Build history of the part. All positions in model axes, mm. Face numbers are marked on the shaded views. A direction names the side the tool comes from. Round coordinates to 2 decimals unless told otherwise and drop trailing zeros. Write each loop counter-clockwise with the first axis right and the second up, starting at its lowest first coordinate (ties: lowest second). Pieces come first, ordered by that corner, then holes. Notation, with made-up numbers: (76.5, 60) - (83.5, 60) arc R28 cw to (83.5, 87) - close; hole circle Ø7 at (-14, -15). An arc over 180 degrees is marked (long way). Write each question's results on one line, items separated by ' | '.
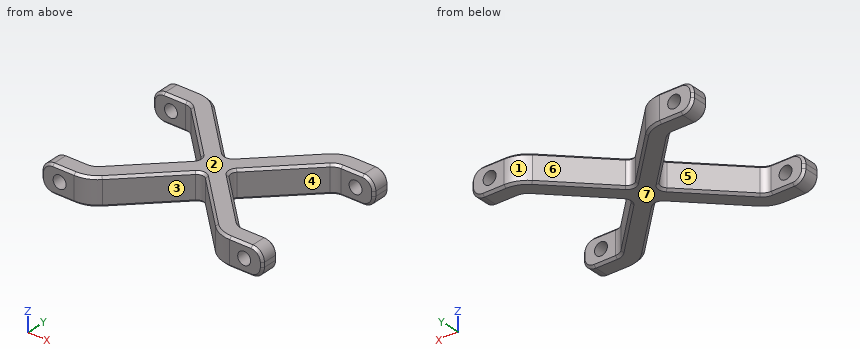
from build123d import *

# Parameters (mm, degrees)
EXTRUIR_L_MINA1_DEPTH    = 6
TALADRO1_D               = 5.6
TALADRO1_DEPTH           = 68
REDONDEO1_R              = 5
REDONDEO1_OF_SIMETR_A1_R = 5
REDONDEO3_R              = 3
CHAFL_N4_SIZE            = 1


# Read off the part's stored shape, not the designer's step: Simetría2
with BuildPart() as part:
    # Croquis1 → Extruir-Lámina1 (new, symmetric)
    with BuildSketch(Plane.XY):
        with BuildLine():
            Line((2.828427125, -2.828427125), (30.192388155, 24.535533906))
            ThreePointArc((30.192388155, 24.535533906), (31.8145049, 25.619397663), (33.727922061, 26))
            Line((33.727922061, 26), (48, 26))
            Line((48, 26), (48, 34))
            Line((48, 34), (33.727922061, 34))
            ThreePointArc((33.727922061, 34), (28.753037441, 33.010433923), (24.535533906, 30.192388155))
            Line((24.535533906, 30.192388155), (-2.828427125, 2.828427125))
            Line((-2.828427125, 2.828427125), (2.828427125, -2.828427125))
        make_face()
    extruir_l_mina1 = extrude(amount=EXTRUIR_L_MINA1_DEPTH, both=True)

    # Taladro1
    with Locations(Plane(origin=(0, 34, 0), x_dir=(1, 0, 0), z_dir=(0, 1, 0))):
        with Locations((40, 0)):
            taladro1 = Hole(TALADRO1_D / 2, depth=TALADRO1_DEPTH)

    # Redondeo1
    redondeo1_edges = [part.edges().sort_by_distance(p)[0] for p in [
        (48, 30, 6),
        (48, 30, -6),
    ]]
    fillet(redondeo1_edges, radius=REDONDEO1_R)

    # Simetría1: Extruir-Lámina1, Taladro1 across plane
    add(extruir_l_mina1.mirror(Plane(origin=(0, 0, 0), x_dir=(0, 0, 1), z_dir=(1, 0, 0))))
    add(taladro1.mirror(Plane(origin=(0, 0, 0), x_dir=(0, 0, 1), z_dir=(1, 0, 0))), mode=Mode.SUBTRACT)

    # Redondeo1 of Simetría1
    redondeo1_of_simetr_a1_edges = [part.edges().sort_by_distance(p)[0] for p in [
        (-48, 30, 6),
        (-48, 30, -6),
    ]]
    fillet(redondeo1_of_simetr_a1_edges, radius=REDONDEO1_OF_SIMETR_A1_R)

    # Simetría2: part across plane


with BuildPart() as part_1:
    add(part.part)
    add(part.part.mirror(Plane.ZX))

    # Redondeo3
    redondeo3_edges = [part_1.edges().sort_by_distance(p)[0] for p in [
        (-5.656854249, 0, 0),
        (5.656854249, 0, 0),
        (0, -5.656854249, 0),
        (0, 5.656854249, 0),
    ]]
    fillet(redondeo3_edges, radius=REDONDEO3_R)

    # Chaflán4
    chafl_n4_edges = [part_1.edges().sort_by_distance(p)[0] for p in [
        (38.363961031, 34, -6),
        (-38.363961031, -26, -6),
        (-31.8145049, -25.619397663, -6),
        (-28.753037441, -33.010433923, 6),
        (-38.363961031, -34, 6),
        (-28.753037441, -33.010433923, -6),
        (-38.363961031, -34, -6),
        (-31.8145049, -25.619397663, 6),
        (-38.363961031, -26, 6),
        (28.753037441, 33.010433923, -6),
        (-48, -26, 0),
        (-46.535533906, -26, 4.535533906),
        (-46.535533906, -26, -4.535533906),
        (-48, -34, 0),
        (-46.535533906, -34, 4.535533906),
        (-46.535533906, -34, -4.535533906),
        (38.363961031, -26, 6),
        (38.363961031, -34, -6),
        (28.753037441, -33.010433923, -6),
        (31.8145049, -25.619397663, 6),
        (31.8145049, -25.619397663, -6),
        (38.363961031, -26, -6),
        (28.753037441, -33.010433923, 6),
        (38.363961031, -34, 6),
        (48, -26, 0),
        (48, -34, 0),
        (38.363961031, 34, 6),
        (46.535533906, -26, 4.535533906),
        (46.535533906, -26, -4.535533906),
        (28.753037441, 33.010433923, 6),
        (46.535533906, -34, 4.535533906),
        (46.535533906, -34, -4.535533906),
        (13.328427125, -18.985281374, 6),
        (13.328427125, -18.985281374, -6),
        (18.985281374, 13.328427125, 6),
        (18.985281374, 13.328427125, -6),
        (18.985281374, -13.328427125, 6),
        (18.985281374, -13.328427125, -6),
        (-18.985281374, 13.328427125, -6),
        (-18.985281374, 13.328427125, 6),
        (-18.985281374, -13.328427125, -6),
        (38.363961031, 26, 6),
        (-18.985281374, -13.328427125, 6),
        (13.328427125, 18.985281374, -6),
        (13.328427125, 18.985281374, 6),
        (-13.328427125, 18.985281374, -6),
        (-13.328427125, -18.985281374, 6),
        (-13.328427125, 18.985281374, 6),
        (0, -6.899494937, -6),
        (0, -6.899494937, 6),
        (31.8145049, 25.619397663, 6),
        (6.899494937, 0, -6),
        (6.899494937, 0, 6),
        (-6.899494937, 0, 6),
        (-6.899494937, 0, -6),
        (0, 6.899494937, 6),
        (0, 6.899494937, -6),
        (-13.328427125, -18.985281374, -6),
        (31.8145049, 25.619397663, -6),
        (38.363961031, 26, -6),
        (48, 26, 0),
        (46.535533906, 26, 4.535533906),
        (46.535533906, 26, -4.535533906),
        (48, 34, 0),
        (46.535533906, 34, 4.535533906),
        (46.535533906, 34, -4.535533906),
        (-31.8145049, 25.619397663, -6),
        (-38.363961031, 26, -6),
        (-28.753037441, 33.010433923, 6),
        (-38.363961031, 34, 6),
        (-38.363961031, 26, 6),
        (-38.363961031, 34, -6),
        (-28.753037441, 33.010433923, -6),
        (-31.8145049, 25.619397663, 6),
        (-48, 26, 0),
        (-48, 34, 0),
        (-46.535533906, 26, 4.535533906),
        (-46.535533906, 26, -4.535533906),
        (-46.535533906, 34, 4.535533906),
        (-46.535533906, 34, -4.535533906),
    ]]
    chamfer(chafl_n4_edges, length=CHAFL_N4_SIZE)


solid = part_1.part
(1) Slice it at A-A, the plane x = 40. Write the cut outline in (y, z).
Worked answers:
outline: (-34, -5) - (-33, -6) - (-27, -6) - (-26, -5) - (-26, -2.8) - (-34, -2.8) - close; (-34, 2.8) - (-26, 2.8) - (-26, 5) - (-27, 6) - (-33, 6) - (-34, 5) - close; (26, -5) - (27, -6) - (33, -6) - (34, -5) - (34, -2.8) - (26, -2.8) - close; (26, 2.8) - (34, 2.8) - (34, 5) - (33, 6) - (27, 6) - (26, 5) - close
(2) Drill centre lines: probe 1 along Z at (x, y) = (-40, 30.75); probe 2 along Y at (x, z) = (36, 4.5); probe 3 along Y at (x, z) = (-24, 0). Where is each one in solid material? Low to high. Write a range as [from, to].
Worked answers:
probe 1: z = [-6, -2.8], [2.8, 6] | probe 2: y = [-34, -26], [26, 34] | probe 3: y = [-29.66, -18.34], [18.34, 29.66]
(3) Slice it at B-B, the plane x = 9. Write the cut outline in (y, z).
Worked answers:
outline: (-14.66, -5) - (-13.24, -6) - (-4.76, -6) - (-3.34, -5) - (-3.34, 5) - (-4.76, 6) - (-13.24, 6) - (-14.66, 5) - close; (3.34, -5) - (4.76, -6) - (13.24, -6) - (14.66, -5) - (14.66, 5) - (13.24, 6) - (4.76, 6) - (3.34, 5) - close
(4) Two-plate mould, pull along Y, no slides. Class the marked faces 4, 5, 6 and 7: released by +Y, released by -Y, zero draft, split by the parting line, or undercut.
Worked answers:
face 4: undercut | face 5: undercut | face 6: released by +Y | face 7: zero draft
(5) Slice it at C-C, the plane z = 0. State how many separate pieces and enclosed holes the cut face has, and give its area (3 significant figures).
Worked answers:
separate pieces: 5 | enclosed holes: 0 | area: 1,680 mm2
(6) Flat gauge pins, fed straight in: pin 1 Ø4 at (y, z) = (1.5, 0) entering from -X; pin 2 Ø1.5 at (x, z) = (-9, -4) entering from +Y; pin 3 Ø5 at (y, z) = (-18, -3) entering from +X; pin 4 Ø4.5 at (x, z) = (-40, 0) entering from -Y. Where does each tip first touch, or does it go through?
Worked answers:
pin 1: stops at x = -9.16 | pin 2: stops at y = 15.41 | pin 3: stops at x = 26.16 | pin 4: passes through
(7) Slice it at D-D, the plane y = -4.5. Write the cut outline in (x, z).
Worked answers:
outline: (-10.16, -5) - (-8.74, -6) - (8.74, -6) - (10.16, -5) - (10.16, 5) - (8.74, 6) - (-8.74, 6) - (-10.16, 5) - close
(8) Tool access for the marked faces 1, 2 and 3: list every direction of +Z, -Z, +X, -X, +Y, -Y with a clear straight run to the whole face (end or side of a thin tool).
Worked answers:
face 1: +Z, -Z, +Y | face 2: +Z, +X, -X, +Y, -Y | face 3: +Z, -Z, -Y
